Geometry: final body of the model. Coordinates: model frame, mm. A direction names the side the tool comes from. Round coordinates to 2 decimals unless told otherwise and drop trailing zeros. Loops run counter-clockwise (first coordinate to the right, second up) from the corner with the lowest first, then second, coordinate; pieces in that order, holes last. Notation, with made-up numbers: (-28.5, 57) - (17.5, 57) arc R16 ccw to (17.5, 80) - close; hole circle Ø3 at (31.5, 10). An arc over 180 degrees is marked (long way). Answer as a JSON object with one key per item and string values. Group by question number.
Item 1: Section D-D (z = 10.25). Return the cut outline in (x, y), plus the area to 3 significant figures.
Item 2: Section C-C (z = 15.5). Return the cut outline in (x, y).
Item 3: Section B-B (x = 22.15). Return the cut outline in (y, z).
Item 4: Line query: line 1 (Y direction, x = -40.5, z = 27.75); line 2 (X direction, y = 13.4, z = 15); line 3 (X direction, y = 12.05, z = 15). Output: solid intervals per line, ascending.
Item 5: Reachability of faces 4 (the face through (0, 12, 0)), 5 (the face through (-49.44, 0.42, 13.8)) from +Z, -Z, +X, -X, +Y, -Y: full face, straight path, thin tool, end or side. Return the list, or none.
Item 6: Section A-A (y = 0). Return the cut outline in (x, z).
Item 7: First-contact query: pin 1 (5.5 mm diameter, centred on x = -39.5, y = -4, fed in from -Z); pin 2 (2.5 mm diameter, centred on x = -22.15, z = 15, fed in from +Y); pin 3 (3 mm diameter, centred on x = -30, z = 4, fed in from -Y); pin 4 (15 mm diameter, centred on x = 35.5, y = 2, fed in from -Z). Flat tips, straight axial feed; report the tip coordinate or a pass-through.
Item 8: Draft query along Z for faces 1 (the face through (-21.14, 13.03, 13.89)), 2 (the face through (1, 14, 30)), 3 (the face through (32.5, -5.75, 13.8)). Return one class per face: released by +Z, released by -Z, zero draft, split by the parting line, or undercut.
```python
from build123d import *

# Parameters (mm, degrees)
SKETCH1_R           = 9.45
BOSS_EXTRUDE1_DEPTH = 30
SKETCH3_R           = 1.5
CUT_EXTRUDE1_DEPTH  = 6
BOSS_EXTRUDE2_START = -2
SKETCH5_R           = 9.45
BOSS_EXTRUDE2_DEPTH = 2


with BuildPart() as part:
    # Sketch1 → Boss-Extrude1 (new body)
    with BuildSketch(Plane.XY):
        with BuildLine():
            Line((-40, 15), (40, 15))
            ThreePointArc((40, 15), (45.476992863, -13.964331319), (29.802327604, 11.00033989))
            Line((29.802327604, 11.00033989), (-29.802327604, 11.00033989))
            ThreePointArc((-29.802327604, 11.00033989), (-45.476992863, -13.964331319), (-40, 15))
        make_face()
        with Locations((-40, 0)):
            Circle(SKETCH1_R, mode=Mode.SUBTRACT)
        with Locations((40, 0)):
            Circle(SKETCH1_R, mode=Mode.SUBTRACT)
    extrude(amount=BOSS_EXTRUDE1_DEPTH)

    # Sketch3 → Cut-Extrude1 (cut)
    with BuildSketch(Plane(origin=(0, 15, 0), x_dir=(1, 0, 0), z_dir=(0, 1, 0))):
        with Locations(Location((-22.15, -15, 0), (0, 0, 270))):
            Circle(SKETCH3_R)
        with Locations(Location((22.15, -15, 0), (0, 0, 270))):
            Circle(SKETCH3_R)
    extrude(amount=-CUT_EXTRUDE1_DEPTH, mode=Mode.SUBTRACT)

    # Sketch5 → Boss-Extrude2 (add)
    with BuildSketch(Plane.XY.offset(30).offset(BOSS_EXTRUDE2_START)):
        with Locations((-40, 0)):
            Circle(SKETCH5_R)
        with Locations((40, 0)):
            Circle(SKETCH5_R)
    extrude(amount=BOSS_EXTRUDE2_DEPTH)


solid = part.part
```
Values:
{
 "1": {"outline": "(-40, 15) arc R15 ccw (long way) to (-29.8, 11) - (29.8, 11) arc R15 ccw (long way) to (40, 15) - close; hole circle Ø18.9 at (-40, 0); hole circle Ø18.9 at (40, 0)", "area": "1,120 mm^2"},
 "2": {"outline": "(-40, 15) arc R15 ccw (long way) to (-29.8, 11) - (-23.56, 11) - (-23.56, 15) - close; (-20.74, 11) - (20.74, 11) - (20.74, 15) - (-20.74, 15) - close; (23.56, 11) - (29.8, 11) arc R15 ccw (long way) to (40, 15) - (23.56, 15) - close; hole circle Ø18.9 at (-40, 0); hole circle Ø18.9 at (40, 0)"},
 "3": {"outline": "(11, 0) - (15, 0) - (15, 13.5) - (11, 13.5) - close; (11, 16.5) - (15, 16.5) - (15, 30) - (11, 30) - close"},
 "4": {"line 1": "y = -14.99 to -9.44, 9.44 to 14.99", "line 2": "x = -46.74 to -23.65, -20.65 to 20.65, 23.65 to 46.74", "line 3": "x = -48.93 to -23.65, -20.65 to 20.65, 23.65 to 48.93"},
 "5": {"face 4": "-Z, +X, -X, +Y, -Y", "face 5": "-Z"},
 "6": {"outline": "(-55, 0) - (-49.45, 0) - (-49.45, 28) - (-30.55, 28) - (-30.55, 0) - (-25, 0) - (-25, 30) - (-55, 30) - close; (25, 0) - (30.55, 0) - (30.55, 28) - (49.45, 28) - (49.45, 0) - (55, 0) - (55, 30) - (25, 30) - close"},
 "7": {"pin 1": "stops at z = 28", "pin 2": "passes through", "pin 3": "stops at y = -12.36", "pin 4": "stops at z = 0"},
 "8": {"face 1": "undercut", "face 2": "released by +Z", "face 3": "zero draft"}
}
